Verification items for the finished model (mm, model axes). Give positions to 0.01 mm unless a question says otherwise; leave off trailing zeros. Order: outer loops, then holes, each group sorted by start corner. A loop starts at its lowest first (then second) coordinate and runs counter-clockwise, first axis right, second up. Notation, with made-up numbers: (66, 87.25) -> (114, 87.25) arc R32 cw to (114, 122.25) -> close; hole circle Ø2 at (-19, 79.5). An arc over 180 degrees is marked (long way). One line per question, with ' | ' between items. Start each with the question number.
Q1. Material ranges on probe 1 along Z at (x, y) = (0, 1.95); probe 2 along Z at (x, y) = (-5.25, 6); probe 3 along X at (y, z) = (14.5, 3), recorded low to high. Write a range as [from, to].
Q2. Section check C-C on y = 4. Record the cut outline in (x, z), plus the area to 3 significant figures.
Q3. Go/stop test with flat-tipped pins: pin 1 (1 mm diameter, centred on x = -11.5, y = 13.5, fed in from +Z); pin 2 (1.2 mm diameter, centred on x = 0, z = -0.5, fed in from -Y); pin 3 (5 mm diameter, centred on y = 5.5, z = 10, fed in from +X). Record where each tip stops, or that it passes through.
Q4. Section check A-A on x = 0. Record the cut outline in (y, z).
Q5. Mould release check, pull along Z, two halves, no side actions. Record for faces 1 (the flat face through (0, 5.5, 0)), 2 (the flat face through (3, 0, 0)), 3 (the flat face through (0, 3, 1)), 4 (the cylindrical face through (-14.985, 7.395, 0.66)): released by +Z, released by -Z, zero draft, split by the parting line, or undercut.
Q6. Section check B-B on z = -1. Record the cut outline in (x, y), plus the area to 3 significant figures.
Q7. Section check D-D on y = 13. Record the cut outline in (x, z).
from build123d import *

# Parameters (mm, degrees)
F0_R     = 15
F1_DEPTH = 15
F3_DEPTH = 5.5


with BuildPart() as f1:
    # F0 (on Front) → F1 (new body)
    with BuildSketch(Plane.XZ):
        Circle(F0_R)
    extrude(amount=-F1_DEPTH)

    # F2 (on face) → F3 (cut)
    with BuildSketch(Plane.XZ):
        with BuildLine():
            ThreePointArc((-1.05, 1), (-0.538516, -1.346291), (1.45, 0))
            ThreePointArc((1.45, 0), (1.346291, 0.538516), (1.05, 1))
            Line((1.05, 1), (-1.05, 1))
        make_face()
    extrude(amount=-F3_DEPTH, mode=Mode.SUBTRACT)


solid = f1.part
Filled in:
1) probe 1: [-15, -1.45], [1, 15] | probe 2: [-14.05, 14.05] | probe 3: [-14.7, 14.7]
2) outline: circle Ø30 at (0, 0); hole (-1.05, 1) arc R1.45 ccw (long way) to (1.45, 0) arc R1.45 ccw to (1.05, 1) -> close | area: 701 mm²
3) pin 1: z = 10.2 | pin 2: y = 5.5 | pin 3: x = 12.99
4) outline: (0, -15) -> (15, -15) -> (15, 15) -> (0, 15) -> (0, 1) -> (5.5, 1) -> (5.5, -1.45) -> (0, -1.45) -> close
5) face 1: undercut | face 2: zero draft | face 3: undercut | face 4: split by the parting line
6) outline: (-14.97, 0) -> (-1.05, 0) -> (-1.05, 5.5) -> (1.05, 5.5) -> (1.05, 0) -> (14.97, 0) -> (14.97, 15) -> (-14.97, 15) -> close | area: 437 mm²
7) outline: circle Ø30 at (0, 0)
